For this review, take the finished solid that the model builds, in its own axes (mm). A direction names the side the tool comes from. Round coordinates to 2 decimals unless told otherwise and drop trailing zeros. One line per question, with ' | ' between items.
```python
from build123d import *

# Parameters (mm, degrees)
F0_R     = 3
F0_R_2   = 2.5
F1_DEPTH = 550
F2_R     = 2
F3_R     = 7


# Not quite as in the source:
# - a feature names something its author has since deleted; it is built from what else it names


with BuildPart() as f1:
    # F0 (on Top) → F1 (new body)
    with BuildSketch(Plane.XY):
        with BuildLine():
            Line((18.15, -30), (30, -30))
            Line((30, -30), (30, -18.15))
            Line((30, -18.15), (27.5, -18.15))
            Line((27.5, -18.15), (27.5, -20.15))
            Line((27.5, -20.15), (21.5477069044, -20.15))
            ThreePointArc((21.5477069044, -20.15), (19.5, -15), (21.5477069044, -9.85))
            Line((21.5477069044, -9.85), (27.5, -9.85))
            Line((27.5, -9.85), (27.5, -11.85))
            Line((27.5, -11.85), (30, -11.85))
            Line((30, -11.85), (30, 11.85))
            Line((30, 11.85), (27.5, 11.85))
            Line((27.5, 11.85), (27.5, 9.85))
            Line((27.5, 9.85), (21.5477069044, 9.85))
            ThreePointArc((21.5477069044, 9.85), (19.5, 15), (21.5477069044, 20.15))
            Line((21.5477069044, 20.15), (27.5, 20.15))
            Line((27.5, 20.15), (27.5, 18.15))
            Line((27.5, 18.15), (30, 18.15))
            Line((30, 18.15), (30, 30))
            Line((30, 30), (18.15, 30))
            Line((18.15, 30), (18.15, 27.5))
            Line((18.15, 27.5), (20.15, 27.5))
            Line((20.15, 27.5), (20.15, 21.5477069044))
            ThreePointArc((20.15, 21.5477069044), (15, 19.5), (9.85, 21.5477069044))
            Line((9.85, 21.5477069044), (9.85, 27.5))
            Line((9.85, 27.5), (11.85, 27.5))
            Line((11.85, 27.5), (11.85, 30))
            Line((11.85, 30), (-11.85, 30))
            Line((-11.85, 30), (-11.85, 27.5))
            Line((-11.85, 27.5), (-9.85, 27.5))
            Line((-9.85, 27.5), (-9.85, 21.5477069044))
            ThreePointArc((-9.85, 21.5477069044), (-15, 19.5), (-20.15, 21.5477069044))
            Line((-20.15, 21.5477069044), (-20.15, 27.5))
            Line((-20.15, 27.5), (-18.15, 27.5))
            Line((-18.15, 27.5), (-18.15, 30))
            Line((-18.15, 30), (-30, 30))
            Line((-30, 30), (-30, 18.15))
            Line((-30, 18.15), (-27.5, 18.15))
            Line((-27.5, 18.15), (-27.5, 20.15))
            Line((-27.5, 20.15), (-21.5477069044, 20.15))
            ThreePointArc((-21.5477069044, 20.15), (-19.5, 15), (-21.5477069044, 9.85))
            Line((-21.5477069044, 9.85), (-27.5, 9.85))
            Line((-27.5, 9.85), (-27.5, 11.85))
            Line((-27.5, 11.85), (-30, 11.85))
            Line((-30, 11.85), (-30, -11.85))
            Line((-30, -11.85), (-27.5, -11.85))
            Line((-27.5, -11.85), (-27.5, -9.85))
            Line((-27.5, -9.85), (-21.5477069044, -9.85))
            ThreePointArc((-21.5477069044, -9.85), (-19.5, -15), (-21.5477069044, -20.15))
            Line((-21.5477069044, -20.15), (-27.5, -20.15))
            Line((-27.5, -20.15), (-27.5, -18.15))
            Line((-27.5, -18.15), (-30, -18.15))
            Line((-30, -18.15), (-30, -30))
            Line((-30, -30), (-18.15, -30))
            Line((-18.15, -30), (-18.15, -27.5))
            Line((-18.15, -27.5), (-20.15, -27.5))
            Line((-20.15, -27.5), (-20.15, -21.5477069044))
            ThreePointArc((-20.15, -21.5477069044), (-15, -19.5), (-9.85, -21.5477069044))
            Line((-9.85, -21.5477069044), (-9.85, -27.5))
            Line((-9.85, -27.5), (-11.85, -27.5))
            Line((-11.85, -27.5), (-11.85, -30))
            Line((-11.85, -30), (11.85, -30))
            Line((11.85, -30), (11.85, -27.5))
            Line((11.85, -27.5), (9.85, -27.5))
            Line((9.85, -27.5), (9.85, -21.5477069044))
            ThreePointArc((9.85, -21.5477069044), (15, -19.5), (20.15, -21.5477069044))
            Line((20.15, -21.5477069044), (20.15, -27.5))
            Line((20.15, -27.5), (18.15, -27.5))
            Line((18.15, -27.5), (18.15, -30))
        make_face()
        with Locations((-25, -25)):
            Circle(F0_R, mode=Mode.SUBTRACT)
        with Locations((-15, -15)):
            Circle(F0_R_2, mode=Mode.SUBTRACT)
        with Locations((25, -25)):
            Circle(F0_R, mode=Mode.SUBTRACT)
        with Locations((15, -15)):
            Circle(F0_R_2, mode=Mode.SUBTRACT)
        with Locations((-25, 25)):
            Circle(F0_R, mode=Mode.SUBTRACT)
        with Locations((-15, 15)):
            Circle(F0_R_2, mode=Mode.SUBTRACT)
        Polygon((-7, 22), (-7, 27.5), (0, 27.5), (7, 27.5), (7, 22), (10, 16), (10, 10), (16, 10), (22, 7), (27.5, 7), (27.5, 0), (27.5, -7), (22, -7), (16, -10), (10, -10), (10, -16), (7, -22), (7, -27.5), (0, -27.5), (-7, -27.5), (-7, -22), (-10, -16), (-10, -10), (-16, -10), (-22, -7), (-27.5, -7), (-27.5, 0), (-27.5, 7), (-22, 7), (-16, 10), (-10, 10), (-10, 16), align=None, mode=Mode.SUBTRACT)
        with Locations((15, 15)):
            Circle(F0_R_2, mode=Mode.SUBTRACT)
        with Locations((25, 25)):
            Circle(F0_R, mode=Mode.SUBTRACT)
    extrude(amount=F1_DEPTH)

    # F2
    f2_edges = [f1.edges().sort_by_distance(p)[0] for p in [
        (-7, 27.5, 275),
        (7, 27.5, 275),
    ]]
    fillet(f2_edges, radius=F2_R)

    # F3
    f3_edges = [f1.edges().sort_by_distance(p)[0] for p in [
        (-10, 16, 275),
        (10, 16, 275),
    ]]
    fillet(f3_edges, radius=F3_R)


solid = f1.part
```
(1) For faces 1 (the flat face through (11, -11, 0)), 2 (the cylindrical face through (19.5, -15.1, 271.2)), list the 3-axis set-ups (+Z, -Z, +X, -X, +Y, -Y) from which the entire face can be reached by the end or side of a thin tool; tool diameter is ignored.
Output values:
face 1: -Z, +X, -X, +Y, -Y | face 2: +Z, -Z
(2) We need section A-A on z = 413. Give the number of separate pieces and of enclosed holes in the cut face, plus the area to 3 significant figures.
Output values:
separate pieces: 1 | enclosed holes: 9 | area: 1,080 mm^2
(3) Insertion check: pin 1 (10 mm diameter, centred on x = 16, z = 174.5, fed in from +Y); pin 2 (4 mm diameter, centred on x = -3.5, y = 21.5, fed in from -Z). Each pin has a flat end and moves straight along its axis. Give the tip position at first contact, or say it passes through.
Output values:
pin 1: y = 30 | pin 2: through
(4) Mouldability with a two-part tool opening along X and no side actions: class faces 3 (the flat face through (0, -27.5, 271)), 4 (the cylindrical face through (15.1, 19.5, 271.2)), 5 (the flat face through (-30, -24, 271)), 6 (the flat face through (0, 30, 271)) as released by +X, released by -X, zero draft, split by the parting line, or undercut.
Output values:
face 3: undercut | face 4: undercut | face 5: released by -X | face 6: zero draft
(5) For probe 1 along Y at (x, z) = (15, 171.5); probe 2 along Y at (x, z) = (1, 374); probe 3 along Y at (x, z) = (15.5, 225), list the stretches that pass through material, from the lowest coordinate up. Write a range as [from, to].
Output values:
probe 1: [-19.5, -17.5], [-12.5, -10], [10, 12.5], [17.5, 19.5] | probe 2: [-30, -27.5], [27.5, 30] | probe 3: [-19.52, -17.45], [-12.55, -10], [10, 12.55], [17.45, 19.52]
